Answer from the drawing. Dimensions are ordinates in mm from the lowest x, y and z of the part. Round coordinates to 2 decimals unless told otherwise and drop trailing zeros. Write each loop counter-clockwise with the first axis right and the second up, starting at its lowest first coordinate (ties: lowest second). Pieces come first, ordered by that corner, then holes. Notation, with made-up numbers: (49.25, 73.5) - (88.25, 73.5) arc R19 ccw to (88.25, 98.5) - close; hole circle Ø7 at (-11, 54.25). An arc over 180 degrees is marked (long way). One line per item, written item: value. Start each with the question number.
(1) A cutting plane is placed at C-C, the plane z = 11.5. Determine the outline of the cut face in (x, y), plus the area to 3 significant figures.
(2) Flat-ended cylindrical pins translate along their axes: pin 1 Ø4 at (y, z) = (19.5, 7.5) entering from -X; pin 2 Ø1 at (x, y) = (43, 22.5) entering from -Z. Find the tip coordinate at first contact, or state that the pin passes through.
(3) Find the intervals of material crossed by L1, parallel to Y at x = 30, z = 31; L2, parallel to X at y = 27.5, z = 40; L3, parallel to Z at x = 25, y = 9.5, in increasing order.
(4) The mould has two halves that part along Y. Classify the marked faces 1, 2, 3 and 4: +Y half, -Y half, draft (parallel to the pull), parting line (faces both ways), or undercut.
(5) A cutting plane is placed at D-D, the plane x = 21. Determine the outline of the cut face in (y, z), plus the area to 3 significant figures.
(6) A cutting plane is placed at A-A, the plane x = 30. Determine the outline of the cut face in (y, z).
(7) A cutting plane is placed at B-B, the plane y = 27.5. Determine the outline of the cut face in (x, z).
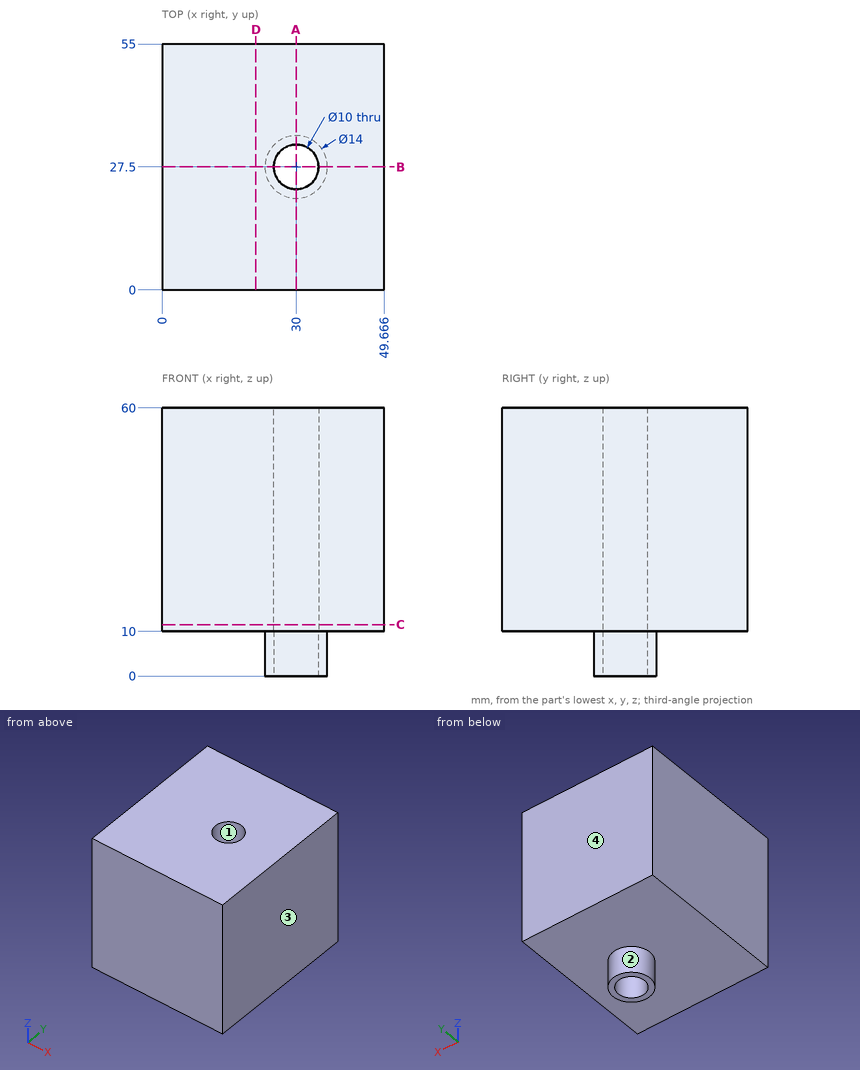
Here are the results:
1. outline: (0, 0) - (49.67, 0) - (49.67, 55) - (0, 55) - close; hole circle Ø10 at (30, 27.5)
1. area: 2,650 mm²
2. pin 1: x = 26.39
2. pin 2: z = 10
3. L1: 0 to 22.5, 32.5 to 55
3. L2: 0 to 25, 35 to 49.67
3. L3: 10 to 60
4. face 1: undercut
4. face 2: parting line
4. face 3: draft
4. face 4: +Y half
5. outline: (0, 10) - (55, 10) - (55, 60) - (0, 60) - close
5. area: 2,750 mm²
6. outline: (0, 10) - (20.5, 10) - (20.5, 0) - (22.5, 0) - (22.5, 60) - (0, 60) - close; (32.5, 0) - (34.5, 0) - (34.5, 10) - (55, 10) - (55, 60) - (32.5, 60) - close
7. outline: (0, 10) - (23, 10) - (23, 0) - (25, 0) - (25, 60) - (0, 60) - close; (35, 0) - (37, 0) - (37, 10) - (49.67, 10) - (49.67, 60) - (35, 60) - close
